Could you check a few things on this model? Use its own coordinates, in mm. A direction names the side the tool comes from. Round coordinates to 2 decimals unless told otherwise and drop trailing zeros. Loops run counter-clockwise (first coordinate to the right, second up) from the corner with the lowest first, then second, coordinate; pieces in that order, holes last. Notation, with made-up numbers: (33, 22) - (46, 22) arc R18 cw to (46, 34) - close; hole circle Ø9 at (-35, 10). An arc over 180 degrees is marked (long way). Answer as CSV lines item,"result". Start each with the question number.
1) Please list where these lines run through material, in increasing order: line 1 along X through (y, z) = (17.5, 16); line 2 along Z through (x, y) = (9.25, 16.5); line 3 along Y through (x, z) = (-1.5, 4).
2) Suppose I cut it at B-B, the plane z = -15. Count the separate pieces of the cut face and the enclosed holes in it, then the cut area to 3 significant figures.
3) I'm going to push flat-ended pins straight in: pin 1 Ø2 at (x, z) = (0.5, 10.5) entering from -Y; pin 2 Ø5 at (y, z) = (0, 0) entering from -X; pin 3 Ø2 at (x, z) = (4, 9) entering from -Y; pin 4 Ø1.5 at (y, z) = (-9, -17.5) entering from +X. Where does each tip first touch, or does it pass through?
4) Suppose I cut it at A-A, the plane x = 3.75. Write out the boundary of the cut face in (y, z), then the cut area to 3 significant figures.
5) Which directions (+Z, -Z, +X, -X, +Y, -Y) give clear straight access to the entire face, cutting with the end or side of a thin tool? Please do faces 3 (the face through (4.521, 22.804, -2.994)), 4 (the face through (2, 2.3, 0)).
6) Suppose I cut it at D-D, the plane x = -6.75. Write out the boundary of the cut face in (y, z), then the cut area to 3 significant figures.
7) We'd pull the mould along Z, two halves only. Please class faces 1 (the face through (0.14, 11.291, -7.616)), 2 (the face through (8.986, 7.509, -23.846)): pulls with the +Z half, pulls with the -Z half, needs draft (parallel to the pull), parting line crosses it, or undercut.
```python
from build123d import *

# Parameters (mm, degrees)
BASE_DEPTH          = 10
BASE_DEPTH_BACK     = 10
ESQUISSE1_R         = 25
ESQUISSE2_R         = 25
ESQUISSE2_R_2       = 23
VIDE_GORGE_DEPTH    = 7
VIDE_JANTE_DEPTH    = 20
ESQUISSE6_R         = 3
VIDE_BLOC_AXE_DEPTH = 4
CHAN_SIZE           = 2


with BuildPart() as part:
    # Esquisse1 → BASE (new, two sides: drawn at the far end of the back side and taken through both)
    with BuildSketch(Plane(origin=(0, 0, 0), x_dir=(0, 0, -1), z_dir=(1, 0, 0)).offset(-BASE_DEPTH_BACK)):
        Circle(ESQUISSE1_R)
        with BuildLine():
            Line((-1.596871942, 2.3), (1.596871942, 2.3))
            ThreePointArc((1.596871942, 2.3), (0, -2.8), (-1.596871942, 2.3))
        make_face(mode=Mode.SUBTRACT)
    extrude(amount=BASE_DEPTH + BASE_DEPTH_BACK)

    # Esquisse2 → VIDE GORGE (cut)
    with BuildSketch(Plane.ZY.offset(8)):
        with Locations(Location((0, 0, 0), (0, 0, 180))):
            Circle(ESQUISSE2_R)
        Circle(ESQUISSE2_R_2, mode=Mode.SUBTRACT)
    vide_gorge = extrude(amount=-VIDE_GORGE_DEPTH, mode=Mode.SUBTRACT)

    # SYM GORGE: VIDE GORGE across plane
    add(vide_gorge.mirror(Plane(origin=(0, 0, 0), x_dir=(0, 0, 1), z_dir=(1, 0, 0))), mode=Mode.SUBTRACT)

    # Esquisse4 → VIDE JANTE (cut)
    with BuildSketch(Plane(origin=(10, 0, 0), x_dir=(0, 0, -1), z_dir=(1, 0, 0))):
        with BuildLine():
            Line((-22, 0), (-5, 0))
            ThreePointArc((-5, 0), (-4.924038765, 0.868240888), (-4.698463104, 1.710100717))
            Line((-4.698463104, 1.710100717), (-20.673237657, 7.524443153))
            ThreePointArc((-20.673237657, 7.524443153), (-21.665770566, 3.820259909), (-22, 0))
        make_face()
        with BuildLine():
            ThreePointArc((-4.698463104, -1.710100717), (-4.924038765, -0.868240888), (-5, 0))
            Line((-5, 0), (-22, 0))
            ThreePointArc((-22, 0), (-21.665770566, -3.820259909), (-20.673237657, -7.524443153))
            Line((-20.673237657, -7.524443153), (-4.698463104, -1.710100717))
        make_face()
        with BuildLine():
            Line((-13.544552457, 17.336236579), (-3.078307377, 3.940053768))
            ThreePointArc((-3.078307377, 3.940053768), (-1.545084972, 4.755282581), (0.174497484, 4.996954135))
            Line((0.174497484, 4.996954135), (0.767788927, 21.986598194))
            ThreePointArc((0.767788927, 21.986598194), (-6.798373876, 20.923243358), (-13.544552457, 17.336236579))
        make_face()
        with BuildLine():
            Line((12.302243876, 18.238826596), (2.795964517, 4.145187863))
            ThreePointArc((2.795964517, 4.145187863), (4.045084972, 2.938926261), (4.80630848, 1.378186779))
            Line((4.80630848, 1.378186779), (21.147757311, 6.064021828))
            ThreePointArc((21.147757311, 6.064021828), (17.798373876, 12.93127555), (12.302243876, 18.238826596))
        make_face()
        with BuildLine():
            ThreePointArc((4.80630848, -1.378186779), (4.045084972, -2.938926261), (2.795964517, -4.145187863))
            Line((2.795964517, -4.145187863), (12.302243876, -18.238826596))
            ThreePointArc((12.302243876, -18.238826596), (17.798373876, -12.93127555), (21.147757311, -6.064021828))
            Line((21.147757311, -6.064021828), (4.80630848, -1.378186779))
        make_face()
        with BuildLine():
            ThreePointArc((0.174497484, -4.996954135), (-1.545084972, -4.755282581), (-3.078307377, -3.940053768))
            Line((-3.078307377, -3.940053768), (-13.544552457, -17.336236579))
            ThreePointArc((-13.544552457, -17.336236579), (-6.798373876, -20.923243358), (0.767788927, -21.986598194))
            Line((0.767788927, -21.986598194), (0.174497484, -4.996954135))
        make_face()
    extrude(amount=-VIDE_JANTE_DEPTH, mode=Mode.SUBTRACT)

    # Esquisse6 → VIDE BLOC AXE (cut)
    with BuildSketch(Plane.ZY.offset(10)):
        Circle(ESQUISSE6_R)
    extrude(amount=-VIDE_BLOC_AXE_DEPTH, mode=Mode.SUBTRACT)

    # CHAN
    chan_edges = [part.edges().sort_by_distance(p)[0] for p in [
        (-1, 0, -23),
        (-8, 0, -23),
        (8, 0, -23),
        (1, 0, -23),
    ]]
    chamfer(chan_edges, length=CHAN_SIZE - 0.0001)  # a hair under: the kernel refuses the full size


solid = part.part
```
Filled sheet:
1,line 1,"-10 to -6.71, -2.29 to 2.29, 6.71 to 10"
1,line 2,"-18.78 to -14.55, -11.13 to -0.58, 12.89 to 18.78"
1,line 3,"-24.17 to -21.63, -5.12 to 5.12, 21.63 to 24.17"
2,separate pieces,"3"
2,enclosed holes,"0"
2,area,"277 mm²"
3,pin 1,"y = -23.12"
3,pin 2,"x = -6"
3,pin 3,"y = -21.56"
3,pin 4,"through"
4,outline,"circle Ø46 at (0, 0); hole (-21.99, -0.77) - (-5, -0.17) arc R5 cw to (-3.94, 3.08) - (-17.34, 13.54) arc R22 ccw to start; hole (-18.24, -12.3) arc R22 ccw to (-6.06, -21.15) - (-1.38, -4.81) arc R5 cw to (-4.15, -2.8) - close; hole (-7.52, 20.67) - (-1.71, 4.7) arc R5 cw to (1.71, 4.7) - (7.52, 20.67) arc R22 ccw to start; hole (1.38, -4.81) - (6.06, -21.15) arc R22 ccw to (18.24, -12.3) - (4.15, -2.8) arc R5 cw to start; hole (2.3, -1.6) - (2.3, 1.6) arc R2.8 ccw (long way) to start; hole (3.94, 3.08) arc R5 cw to (5, -0.17) - (21.99, -0.77) arc R22 ccw to (17.34, 13.54) - close"
4,area,"837 mm²"
5,face 3,"none"
5,face 4,"+X, -X"
6,outline,"circle Ø47.5 at (0, 0); hole (-21.99, -0.77) - (-5, -0.17) arc R5 cw to (-3.94, 3.08) - (-17.34, 13.54) arc R22 ccw to start; hole (-18.24, -12.3) arc R22 ccw to (-6.06, -21.15) - (-1.38, -4.81) arc R5 cw to (-4.15, -2.8) - close; hole (-7.52, 20.67) - (-1.71, 4.7) arc R5 cw to (1.71, 4.7) - (7.52, 20.67) arc R22 ccw to start; hole circle Ø6 at (0, 0); hole (1.38, -4.81) - (6.06, -21.15) arc R22 ccw to (18.24, -12.3) - (4.15, -2.8) arc R5 cw to start; hole (3.94, 3.08) arc R5 cw to (5, -0.17) - (21.99, -0.77) arc R22 ccw to (17.34, 13.54) - close"
6,area,"943 mm²"
7,face 1,"undercut"
7,face 2,"parting line crosses it"
